Input: dimensioned drawing with shaded views. Units: mm. Origin: part minimum x, y, z. A direction names the side the tool comes from. Round coordinates to 2 decimals unless told otherwise and drop trailing zeros. Loops run counter-clockwise (first coordinate to the right, second up) from the corner with the lowest first, then second, coordinate; pieces in that order, holes last. Notation, with made-up numbers: (-13, 80) - (36, 80) arc R22 ccw to (36, 118) - close; hole circle Ø11 at (43, 82). An arc over 180 degrees is marked (long way). Write each question's results on one line, items separated by ' | '.
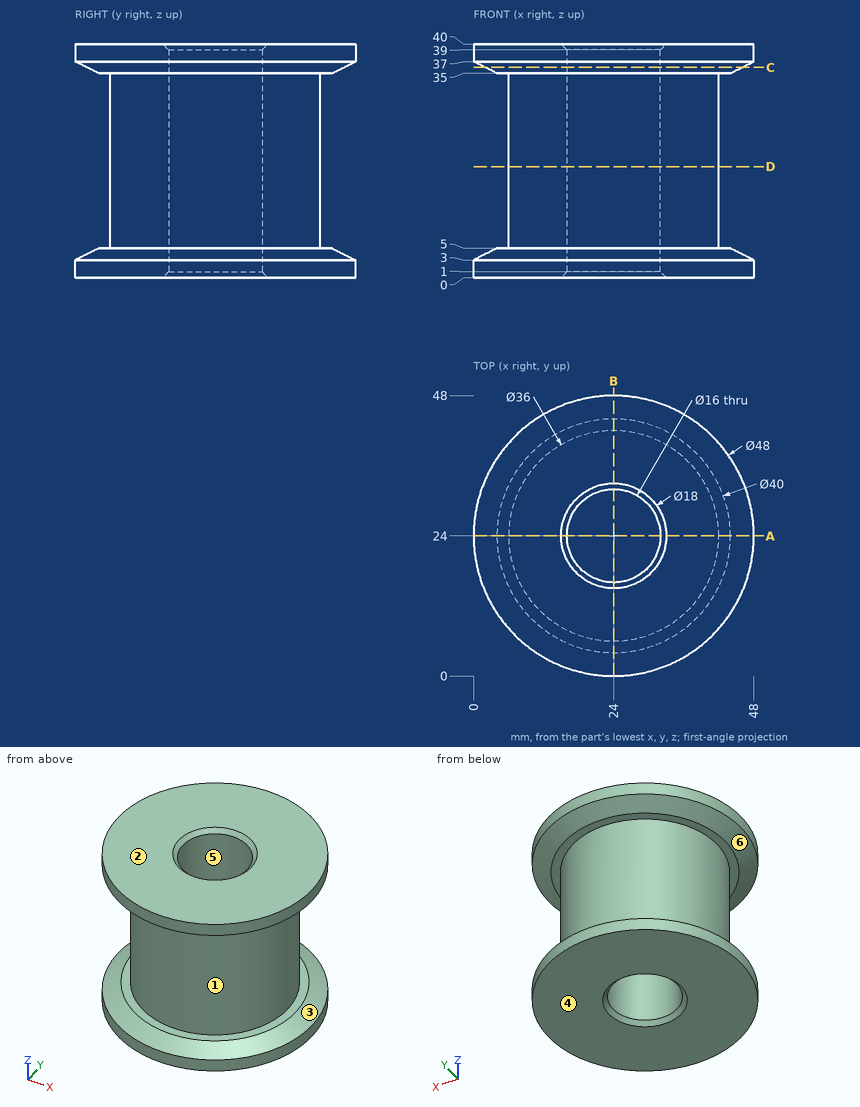
1. Section query C-C, the plane z = 36. Output: boundary loops of the cut face in (x, y), plus the area to 3 significant figures.
Answer:
outline: circle Ø44 at (24, 24); hole circle Ø16 at (24, 24) | area: 1,320 mm^2
2. Section query D-D, the plane z = 19. Output: boundary loops of the cut face in (x, y), plus the area to 3 significant figures.
Answer:
outline: circle Ø36 at (24, 24); hole circle Ø16 at (24, 24) | area: 817 mm^2
3. Section query A-A, the plane y = 24. Output: boundary loops of the cut face in (x, z).
Answer:
outline: (0, 0) - (15, 0) - (16, 1) - (16, 39) - (15, 40) - (0, 40) - (0, 37) - (4, 35) - (6, 35) - (6, 5) - (4, 5) - (0, 3) - close; (32, 1) - (33, 0) - (48, 0) - (48, 3) - (44, 5) - (42, 5) - (42, 35) - (44, 35) - (48, 37) - (48, 40) - (33, 40) - (32, 39) - close
4. Contact query for flat-ended pins moving along their axis: pin 1 (5 mm diameter, centred on y = 23, z = 23, fed in from -X); pin 2 (2 mm diameter, centred on x = 28, z = 28.5, fed in from +Y); pin 3 (12 mm diameter, centred on x = 37.5, z = 28.5, fed in from +Y). Output: stop coordinate, or through.
Answer:
pin 1: x = 6 | pin 2: y = 41.75 | pin 3: y = 40.36
5. Set-up query: the marked faces 5 and 6. Return all of +Z, -Z, +X, -X, +Y, -Y with unobstructed straight access to the full face (end or side cutting, diameter ignored); none if empty.
Answer:
face 5: +Z, -Z | face 6: none
6. Line query: line 1 (Z direction, x = 35.5, y = 39.5); line 2 (Y direction, x = 24, z = 10); line 3 (Z direction, x = 45.5, y = 17). Output: solid intervals per line, ascending. Write a range as [from, to].
Answer:
line 1: [0, 5], [35, 40] | line 2: [6, 16], [32, 42] | line 3: [0, 3.69], [36.31, 40]
7. Mould query, pull axis Z, two halves, no side actions, for the marked faces 1, 2, 3 and 4. Classes: pulls with the +Z half, pulls with the -Z half, needs draft (parallel to the pull), parting line crosses it, or undercut.
Answer:
face 1: undercut | face 2: pulls with the +Z half | face 3: undercut | face 4: pulls with the -Z half
